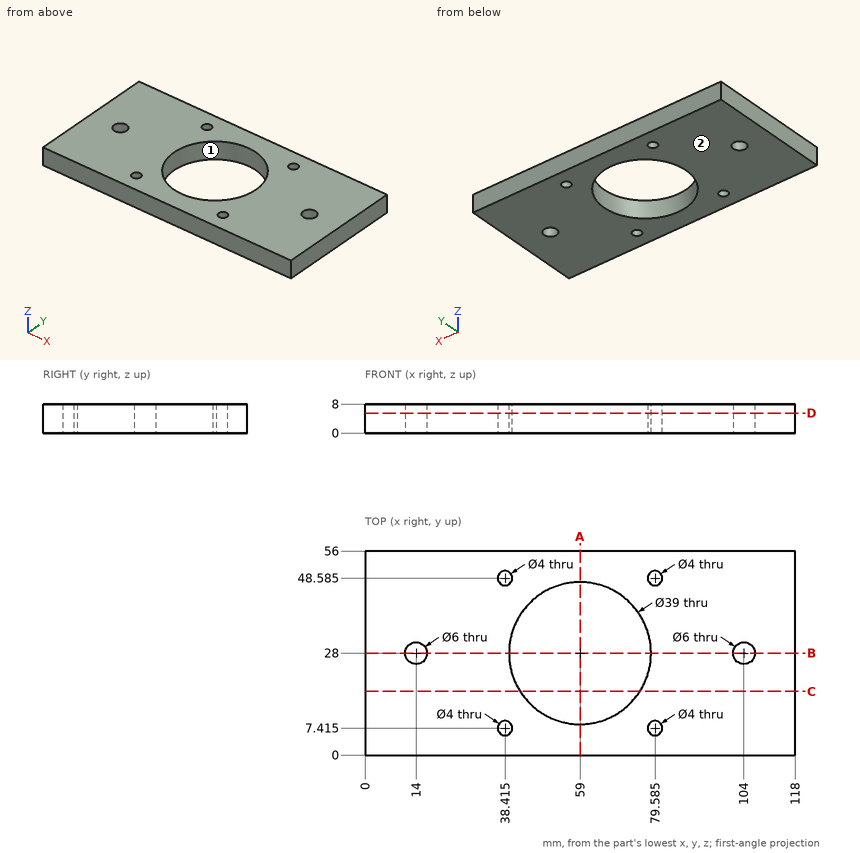
Here's the drawing with two shaded views (mm, measured from the low corner). I have some questions. Coordinates: 2 decimals unless noted, no trailing zeros. Write each loop counter-clockwise with the first axis right and the second up, starting at its lowest first coordinate (ties: lowest second). Pieces come first, ordered by that corner, then holes. Notation, with made-up numbers: M 32,24.25 L 53,24.25 A35 cw 53,60.25 Z; hole C 24.25,42 d8. An arc over 180 degrees is marked long. Answer as CSV lines item,"result". Start each with the question number.
1) I want a section at C-C, the plane y = 17.5. Please give me the cut outline in (x, z), and give its area (3 significant figures).
2) Please list where these lines run through material, in increasing order: line 1 (Y direction, x = 104, z = 2.5); line 2 (Y direction, x = 59, z = 6); line 3 (X direction, y = 10, z = 1). Write a range as from..to.
3) I want a section at B-B, the plane y = 28. Please give me the cut outline in (x, z), and give its area (3 significant figures).
4) I want a section at D-D, the plane z = 5.5. Please give me the cut outline in (x, y) (3 decimals).
5) We'd pull the mould along X, two halves only. Please class the marked faces 1 and 2: +X half, -X half, draft (parallel to the pull), parting line (faces both ways), or undercut.
6) I want a section at A-A, the plane x = 59. Please give me the cut outline in (y, z), and give its area (3 significant figures).
Data:
1,outline,"M 0,0 L 42.57,0 L 42.57,8 L 0,8 Z; M 75.43,0 L 118,0 L 118,8 L 75.43,8 Z"
1,area,"681 mm^2"
2,line 1,"y = 0..25, 31..56"
2,line 2,"y = 0..8.5, 47.5..56"
2,line 3,"x = 0..51.5, 66.5..118"
3,outline,"M 0,0 L 11,0 L 11,8 L 0,8 Z; M 17,0 L 39.5,0 L 39.5,8 L 17,8 Z; M 78.5,0 L 101,0 L 101,8 L 78.5,8 Z; M 107,0 L 118,0 L 118,8 L 107,8 Z"
3,area,"536 mm^2"
4,outline,"M 0,0 L 118,0 L 118,56 L 0,56 Z; hole C 14,28 d6; hole C 38.415,7.415 d4; hole C 38.415,48.585 d4; hole C 59,28 d39; hole C 79.585,7.415 d4; hole C 79.585,48.585 d4; hole C 104,28 d6"
5,face 1,"undercut"
5,face 2,"draft"
6,outline,"M 0,0 L 8.5,0 L 8.5,8 L 0,8 Z; M 47.5,0 L 56,0 L 56,8 L 47.5,8 Z"
6,area,"136 mm^2"
